```python
from build123d import *

# Parameters (mm, degrees)
SKETCH1_R               = 20
SKETCH1_R_2             = 1.65
BOSS_EXTRUDE2_DEPTH     = 3.5
CUT_EXTRUDE1_DEPTH      = 1
CUT_EXTRUDE1_DEPTH_BACK = 4.5
SKETCH4_R               = 6.45
BOSS_EXTRUDE3_DEPTH     = 30
SKETCH5_R               = 5
BOSS_EXTRUDE4_DEPTH     = 2
CUT_EXTRUDE2_START      = -3.5
CUT_EXTRUDE2_DEPTH      = 1.5
SKETCH7_R               = 10.5
SKETCH7_R_2             = 7.5
CUT_EXTRUDE3_DEPTH      = 22.225065807


with BuildPart() as part:
    # Sketch1 → Boss-Extrude2 (new body)
    with BuildSketch(Plane(origin=(0, 0, 0), x_dir=(1, 0, 0), z_dir=(0, 1, 0))):
        with Locations((-12.255661444, 8.620165848)):
            Circle(SKETCH1_R)
        with Locations((-23.755661444, 20.120165848)):
            Circle(SKETCH1_R_2, mode=Mode.SUBTRACT)
        with Locations((-0.755661444, 20.120165848)):
            Circle(SKETCH1_R_2, mode=Mode.SUBTRACT)
        with Locations((-23.755661444, -2.879834152)):
            Circle(SKETCH1_R_2, mode=Mode.SUBTRACT)
        with Locations((-0.755661444, -2.879834152)):
            Circle(SKETCH1_R_2, mode=Mode.SUBTRACT)
    extrude(amount=BOSS_EXTRUDE2_DEPTH)

    # Sketch3 → Cut-Extrude1 (cut, two sides)
    with BuildSketch(Plane(origin=(0, 3.5, 0), x_dir=(1, 0, 0), z_dir=(0, 1, 0))) as cut_extrude1_sk:
        Polygon((-129.974635183, 24.98323402), (-23.755661444, 24.98323402), (-0.755661444, 24.98323402), (105.463312296, 24.98323402), (105.463312296, 237.421181499), (-129.974635183, 237.421181499), align=None)
    extrude(amount=CUT_EXTRUDE1_DEPTH, mode=Mode.SUBTRACT)
    extrude(cut_extrude1_sk.sketch, amount=-CUT_EXTRUDE1_DEPTH_BACK, mode=Mode.SUBTRACT)

    # Sketch4 → Boss-Extrude3 (add)
    with BuildSketch(Plane(origin=(0, 0, -24.98323402), x_dir=(-1, 0, 0), z_dir=(0, 0, -1))):
        with BuildLine():
            Line((4.255661444, 13.225065807), (4.255661444, 3.5))
            Line((4.255661444, 3.5), (20.255661444, 3.5))
            Line((20.255661444, 3.5), (20.255661444, 13.225065807))
            ThreePointArc((20.255661444, 13.225065807), (12.255661444, 21.225065807), (4.255661444, 13.225065807))
        make_face()
        with Locations((12.255661444, 13.225065807)):
            Circle(SKETCH4_R, mode=Mode.SUBTRACT)
    extrude(amount=-BOSS_EXTRUDE3_DEPTH)

    # Sketch5 → Boss-Extrude4 (add)
    with BuildSketch(Plane.XY.offset(5.01676598)):
        with BuildLine():
            Line((-20.255661444, 13.225065807), (-20.255661444, 5))
            Line((-20.255661444, 5), (-4.255661444, 5))
            Line((-4.255661444, 5), (-4.255661444, 13.225065807))
            ThreePointArc((-4.255661444, 13.225065807), (-12.255661444, 21.225065807), (-20.255661444, 13.225065807))
        make_face()
        with Locations((-12.255661444, 13.225065807)):
            Circle(SKETCH5_R, mode=Mode.SUBTRACT)
    extrude(amount=BOSS_EXTRUDE4_DEPTH)

    # Sketch6 → Cut-Extrude2 (cut)
    with BuildSketch(Plane.XZ.offset(CUT_EXTRUDE2_START)):
        Polygon((-22.023610636, -17.120165848), (-25.487712251, -17.120165848), (-27.219763059, -20.120165848), (-25.487712251, -23.120165848), (-22.023610636, -23.120165848), (-20.291559828, -20.120165848), align=None)
        Polygon((-22.023610636, -0.120165848), (-20.291559828, 2.879834152), (-22.023610636, 5.879834152), (-25.487712251, 5.879834152), (-27.219763059, 2.879834152), (-25.487712251, -0.120165848), align=None)
        Polygon((0.976389364, -0.120165848), (2.708440172, 2.879834152), (0.976389364, 5.879834152), (-2.487712251, 5.879834152), (-4.219763059, 2.879834152), (-2.487712251, -0.120165848), align=None)
        Polygon((0.976389364, -17.120165848), (-2.487712251, -17.120165848), (-4.219763059, -20.120165848), (-2.487712251, -23.120165848), (0.976389364, -23.120165848), (2.708440172, -20.120165848), align=None)
    extrude(amount=CUT_EXTRUDE2_DEPTH, mode=Mode.SUBTRACT)

    # Sketch7 → Cut-Extrude3 (cut, through all)
    with BuildSketch(Plane.XZ):
        with Locations((-32.255661444, -8.620165848)):
            Circle(SKETCH7_R)
        with Locations((7.744338556, -8.620165848)):
            Circle(SKETCH7_R)
        with Locations((-12.255661444, 11.379834152)):
            Circle(SKETCH7_R_2)
    extrude(amount=-CUT_EXTRUDE3_DEPTH, mode=Mode.SUBTRACT)


solid = part.part
```
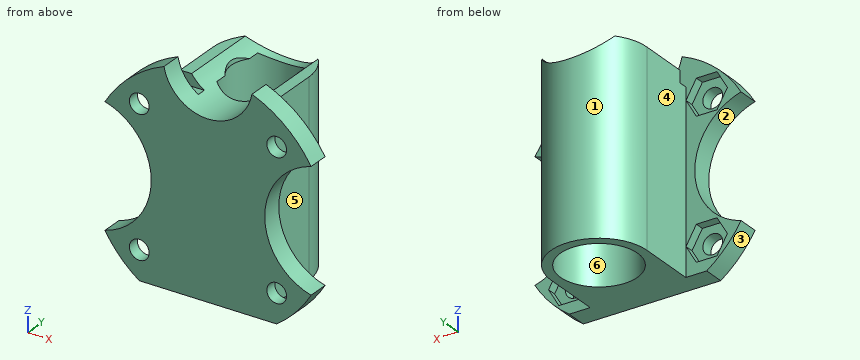
Geometry check sheet. Reference: the model listing, model coordinates, mm. Face numbers are marked on the shaded views. A direction names the side the tool comes from. Give positions to 0.01 mm unless a question says otherwise; leave off trailing zeros. Write each loop counter-clockwise with the first axis right and the second up, starting at its lowest first coordinate (ties: lowest second). Pieces come first, ordered by that corner, then holes.
1) Material ranges on L1, parallel to Y at x = -12, z = -20.5; L2, parallel to Z at x = -3.5, y = 3; L3, parallel to X at y = 2.5, z = 3, recorded low to high.
2) Section check B-B, the plane z = -1.5. Record the boundary of the cut face in (x, y).
3) Section check D-D, the plane y = 4. Record the boundary of the cut face in (x, z).
4) Gauge pin test, flat ends, axial feed: pin 1 (1.2 mm diameter, centred on x = -7, y = 15, fed in from -Z); pin 2 (1 mm diameter, centred on x = -5, y = 13.5, fed in from +Z); pin 3 (1.6 mm diameter, centred on x = -23.5, y = 3, fed in from +Z). Record the tip position at first contact, or that the pin passes through.
5) Release check for a two-part mould opening along Z. For the marked faces 1, 2 and 3 record: pulls with the +Z half, pulls with the -Z half, needs draft (parallel to the pull), parting line crosses it, or undercut.
6) Access from +Z, -Z, +X, -X, +Y, -Y to the whole of each face (thin tool, end or side, straight path). Record for the marked faces 4, 5 and 6.
7) Section check A-A, the plane x = -11. Record the boundary of the cut face in (y, z), and give its area (3 significant figures).
8) Section check C-C, the plane x = -23. Record the boundary of the cut face in (y, z).
Computed:
1. L1: y = 0 to 6.78, 19.67 to 21.22
1. L2: z = -24.98 to -21.37, -18.87 to 1.63, 4.13 to 9.36
1. L3: x = -28.53 to -27.15, -20.36 to -4.15, 2.64 to 4.02
2. outline: (-24.54, 0) - (0.03, 0) - (0.03, 3.5) - (-4.26, 3.5) - (-4.26, 13.23) arc R8 ccw to (-20.26, 13.23) - (-20.26, 3.5) - (-24.54, 3.5) - close; hole circle Ø12.9 at (-12.26, 13.23)
3. outline: (-20.26, -24.98) - (-4.26, -24.98) - (-4.26, 5.02) - (-8.29, 5.02) arc R7.5 cw to (-16.23, 5.02) - (-20.26, 5.02) - close
4. pin 1: stops at z = 5.02
4. pin 2: stops at z = 7.02
4. pin 3: stops at z = 8.44
5. face 1: needs draft
5. face 2: undercut
5. face 3: pulls with the -Z half
6. face 4: +Z, -Z, -X, +Y
6. face 5: +Z, -Z, +X, +Y
6. face 6: -Z
7. outline: (0, -24.98) - (6.9, -24.98) - (6.9, 3.99) - (0, 3.99) - close; (19.55, -24.98) - (21.13, -24.98) - (21.13, 3.99) - (19.55, 3.99) - close
7. area: 245 mm2
8. outline: (0, -24.98) - (3.5, -24.98) - (3.5, -23.12) - (2, -23.12) - (2, -21.59) - (0, -21.59) - close; (0, -18.65) - (2, -18.65) - (2, -17.12) - (3.5, -17.12) - (3.5, -13.58) - (0, -13.58) - close; (0, -3.66) - (3.5, -3.66) - (3.5, -0.12) - (2, -0.12) - (2, 1.41) - (0, 1.41) - close; (0, 4.35) - (2, 4.35) - (2, 5.88) - (3.5, 5.88) - (3.5, 8.25) - (0, 8.25) - close
